Could you check a few things on this model? Use its own coordinates, in mm. A direction names the side the tool comes from. Give positions to 0.01 mm unless a question says otherwise; leave off trailing zeros. Loops run counter-clockwise (first coordinate to the right, second up) from the corner with the lowest first, then second, coordinate; pieces in that order, holes last. Notation, with made-up numbers: M 74.25,28 L 132.25,28 A8 ccw 132.25,38 Z; hole C 87,20.5 d2. An arc over 180 degrees is marked long. Answer in a Markdown table with one row per item. Add a question column.
```python
from build123d import *

# Parameters (mm, degrees)
SKETCH1_W                              = 165.1
SKETCH1_H                              = 157.469327732
BOSS_EXTRUDE1_DEPTH                    = 38.1
BOSS_EXTRUDE1_DEPTH_BACK               = 2
SKETCH2_W                              = 95.25
SKETCH2_H                              = 95.25
BOSS_EXTRUDE2_DEPTH                    = 38.1
BOSS_EXTRUDE3_START                    = -95.25
BOSS_EXTRUDE3_DEPTH                    = 95.25
SKETCH4_R                              = 12.7
CUT_EXTRUDE1_DEPTH                     = 131.175
SKETCH5_W                              = 38.1
SKETCH5_H                              = 85.725
CUT_EXTRUDE3_DEPTH                     = 127.359663866
FILLET1_R                              = 3.175
SKETCH6_R                              = 26
CUT_EXTRUDE4_DEPTH                     = 36.83
SKETCH9_R                              = 76.2
SKETCH9_R_2                            = 69.85
CUT_EXTRUDE5_DEPTH                     = 8
F_1_2_14_NPSM_TAPPED_HOLE1_D           = 18.9738
F_1_2_14_NPSM_TAPPED_HOLE1_DEPTH       = 63.5
F_1_2_14_NPSM_TAPPED_HOLE1_CSINK_D     = 22.1742
F_1_2_14_NPSM_TAPPED_HOLE1_CSINK_ANGLE = 100
F_1_2_14_NPSM_TAPPED_HOLE1_TIP         = 5.700304607
SKETCH16_R                             = 6.35
CUT_EXTRUDE6_DEPTH                     = 25
SKETCH17_R                             = 6.35
CUT_EXTRUDE7_DEPTH                     = 126.825


with BuildPart() as part:
    # Sketch1 → Boss-Extrude1 (new body, two sides)
    with BuildSketch(Plane(origin=(0, 0, 0), x_dir=(1, 0, 0), z_dir=(0, 1, 0))) as boss_extrude1_sk:
        Rectangle(SKETCH1_W, SKETCH1_H)
    extrude(amount=BOSS_EXTRUDE1_DEPTH)
    extrude(boss_extrude1_sk.sketch, amount=-BOSS_EXTRUDE1_DEPTH_BACK)

    # Sketch2 → Boss-Extrude2 (add)
    with BuildSketch(Plane(origin=(0, 38.1, 0), x_dir=(1, 0, 0), z_dir=(0, 1, 0))):
        Rectangle(SKETCH2_W, SKETCH2_H)
    extrude(amount=BOSS_EXTRUDE2_DEPTH)

    # Sketch3 → Boss-Extrude3 (add)
    with BuildSketch(Plane.ZY.offset(47.625).offset(BOSS_EXTRUDE3_START)):
        with BuildLine():
            Line((-47.625, 76.2), (47.625, 76.2))
            ThreePointArc((47.625, 76.2), (0, 123.825), (-47.625, 76.2))
        make_face()
    extrude(amount=BOSS_EXTRUDE3_DEPTH)

    # Sketch4 → Cut-Extrude1 (cut, through all)
    with BuildSketch(Plane.ZY.offset(47.625)):
        with Locations((0, 76.2)):
            Circle(SKETCH4_R)
    extrude(amount=-CUT_EXTRUDE1_DEPTH, mode=Mode.SUBTRACT)

    # Sketch5 → Cut-Extrude3 (cut, through all)
    with BuildSketch(Plane.XY.offset(47.625)):
        with Locations((0, 80.9625)):
            Rectangle(SKETCH5_W, SKETCH5_H)
    extrude(amount=-CUT_EXTRUDE3_DEPTH, mode=Mode.SUBTRACT)

    # Fillet1
    fillet1_edges = [part.edges().sort_by_distance(p)[0] for p in [
        (82.55, 18.05, 78.734663866),
        (-82.55, 18.05, 78.734663866),
        (-82.55, 18.05, -78.734663866),
        (82.55, 18.05, -78.734663866),
    ]]
    fillet(fillet1_edges, radius=FILLET1_R)

    # Sketch6 → Cut-Extrude4 (cut)
    with BuildSketch(Plane.XZ.offset(2)):
        Circle(SKETCH6_R)
    extrude(amount=-CUT_EXTRUDE4_DEPTH, mode=Mode.SUBTRACT)

    # Sketch9 → Cut-Extrude5 (cut)
    with BuildSketch(Plane.XZ.offset(2)):
        Circle(SKETCH9_R)
        Circle(SKETCH9_R_2, mode=Mode.SUBTRACT)
    extrude(amount=-CUT_EXTRUDE5_DEPTH, mode=Mode.SUBTRACT)

    # 1/2-14 NPSM Tapped Hole1
    with Locations(Plane.XY.offset(78.734663866)):
        with Locations((0, 18.05)):
            CounterSinkHole(F_1_2_14_NPSM_TAPPED_HOLE1_D / 2, F_1_2_14_NPSM_TAPPED_HOLE1_CSINK_D / 2, depth=F_1_2_14_NPSM_TAPPED_HOLE1_DEPTH, counter_sink_angle=F_1_2_14_NPSM_TAPPED_HOLE1_CSINK_ANGLE)
            with Locations((0, 0, -(F_1_2_14_NPSM_TAPPED_HOLE1_DEPTH + F_1_2_14_NPSM_TAPPED_HOLE1_TIP / 2))):  # 118° drill point
                Cone(0, F_1_2_14_NPSM_TAPPED_HOLE1_D / 2, F_1_2_14_NPSM_TAPPED_HOLE1_TIP, mode=Mode.SUBTRACT)

    # Sketch16 → Cut-Extrude6 (cut)
    with BuildSketch(Plane.XZ.offset(2)):
        with Locations((0, 46.734663866)):
            Circle(SKETCH16_R)
    extrude(amount=-CUT_EXTRUDE6_DEPTH, mode=Mode.SUBTRACT)

    # Sketch17 → Cut-Extrude7 (cut, through all)
    with BuildSketch(Plane.XZ.offset(2)):
        with Locations((-61.963767235, 61.963767235)):
            Circle(SKETCH17_R)
        with Locations((61.963767235, 61.963767235)):
            Circle(SKETCH17_R)
        with Locations((61.963767235, -61.963767235)):
            Circle(SKETCH17_R)
        with Locations((-61.963767235, -61.963767235)):
            Circle(SKETCH17_R)
    extrude(amount=-CUT_EXTRUDE7_DEPTH, mode=Mode.SUBTRACT)


solid = part.part
```
Item 1: I need wall thicknesses on L1, parallel to Z at x = 0, y = 5.75; L2, parallel to X at y = 10, z = 60.5; L3, parallel to X at y = 42, z = 43 (3 decimals). Which ranges of each line are inside material? Lowest first, please.
Item 2: Suppose I cut it at C-C (z = 0). Give the number of separate pieces and of enclosed holes in the cut face, then the cut area to 3 significant figures.
Item 3: For P1, Ø6, axis at x = -27.5, z = 17.5, coming from the +Y side; P2, Ø15.5, axis at x = -4, z = -5, coming from the -Y side; P3, Ø5, axis at x = 47, z = 35, coming from the +Y side, each with a flat end and sliding along its axis, tell me the tip position at first contact or that it passes through.
Item 4: Suppose I cut it at B-B (x = 0). List the corners of the cut face in (y, z) for me.
Item 5: For faces 5 (the face through (19.05, 90, 1)), 6 (the face through (33, 57, -47.625)), 7 (the face through (60.587, 17.769, 55.765)), 8 (the face through (-34, 57, 47.625)), 9 (the face through (-55.431, 1.944, -42.503)), which set-ups out of +Z, -Z, +X, -X, +Y, -Y let a thin tool reach every point of the face, with its end or its side?
Item 6: If we mould it in two halves opening along X, with no side actions, what happens to faces 1 (the face through (1.235, 27.456, 50.427)), 2 (the face through (47.625, 91, -1)), 3 (the face through (0, 34.83, 0)), 4 (the face through (-62, -2, 46))? For each: +X half, -X half, draft (parallel to the pull), parting line (faces both ways), or undercut.
Item 7: Suppose I cut it at A-A (z = 65.5). List the corners of the cut face in (x, y) for me.
Item 8: Suppose I cut it at D-D (y = 98.5). List the corners of the cut face in (x, z) for me (3 decimals).
Values found:
| question | item | result |
|---|---|---|
| 1 | L1 | -78.73 to -76.2, -69.85 to -26, 26 to 40.38, 53.08 to 69.85, 76.2 to 78.73 |
| 1 | L2 | -82.55 to -68.14, -55.78 to -5.02, 5.02 to 55.78, 68.14 to 82.55 |
| 1 | L3 | -47.625 to -19.05, 19.05 to 47.625 |
| 2 | separate pieces | 3 |
| 2 | enclosed holes | 0 |
| 2 | area | 8,050 mm² |
| 3 | P1 | y = 121.56 |
| 3 | P2 | y = 34.83 |
| 3 | P3 | y = 111.01 |
| 4 | outline | M -2,-78.73 L 38.1,-78.73 L 38.1,78.73 L 29.14,78.73 L 27.54,77.39 L 27.54,26 L 34.83,26 L 34.83,-26 L -2,-26 L -2,-69.85 L 6,-69.85 L 6,-76.2 L -2,-76.2 Z; M -2,26 L 8.56,26 L 8.56,40.38 L -2,40.38 Z; M -2,53.08 L 8.56,53.08 L 8.56,77.39 L 6.96,78.73 L -2,78.73 L -2,76.2 L 6,76.2 L 6,69.85 L -2,69.85 Z |
| 5 | face 5 | +Z, -Z, +Y |
| 5 | face 6 | -Z, +X, -X, +Y |
| 5 | face 7 | +Y, -Y |
| 5 | face 8 | +Z, +X, -X, +Y |
| 5 | face 9 | -Y |
| 6 | face 1 | undercut |
| 6 | face 2 | +X half |
| 6 | face 3 | undercut |
| 6 | face 4 | draft |
| 7 | outline | M -82.55,-2 L -67.24,-2 L -67.24,38.1 L -82.55,38.1 Z; M -56.69,-2 L -38.94,-2 L -38.94,6 L -24.26,6 L -24.26,-2 L 24.26,-2 L 24.26,6 L 38.94,6 L 38.94,-2 L 56.69,-2 L 56.69,38.1 L -56.69,38.1 Z; M 67.24,-2 L 82.55,-2 L 82.55,38.1 L 67.24,38.1 Z; hole C 0,18.05 d18.97 |
| 8 | outline | M -47.625,-42.081 L -19.05,-42.081 L -19.05,42.081 L -47.625,42.081 Z; M 19.05,-42.081 L 47.625,-42.081 L 47.625,42.081 L 19.05,42.081 Z |
